Could you check a few things on this model? Use its own coordinates, in mm. Face numbers are marked on the shaded views. A direction names the side the tool comes from. Coordinates: 2 decimals unless noted, no trailing zeros. Write each loop counter-clockwise with the first axis right and the second up, starting at its lowest first coordinate (ties: lowest second). Pieces come first, ordered by that corner, then holes. Notation, with made-up numbers: (14, 37) - (19, 37) arc R25 cw to (19, 55) - close; hole circle Ø1 at (20, -34). An arc over 180 degrees is marked (long way). Answer as a JSON object with one key per item and string values. Group by question number.
1) Please list where these lines run through material, in increasing order: line 1 along Y through (x, z) = (2.5, 0.25); line 2 along X through (y, z) = (-1.9, -0.3); line 3 along X through (y, z) = (2.1, -1.4).
2) On a 3-axis mill with a long thin cutter (end or side, diameter ignored), from which of +Z, -Z, +X, -X, +Y, -Y can I reach the whole of each face in a straight line? I mean the marked faces 1 and 2. Say none if no direction works.
3) If we section it at A-A (x = 3.5): Write out the boundary of the cut face in (y, z).
4) Will these pins go through, and if not, where does the flat tip stop? pin 1 Ø1 at (x, z) = (3.5, -2) entering from +Y; pin 2 Ø3 at (x, z) = (3.5, 1.5) entering from -Y; pin 3 Ø3 at (x, z) = (3.5, 1) entering from +Y; pin 4 Ø1 at (x, y) = (3, 0) entering from -Z.
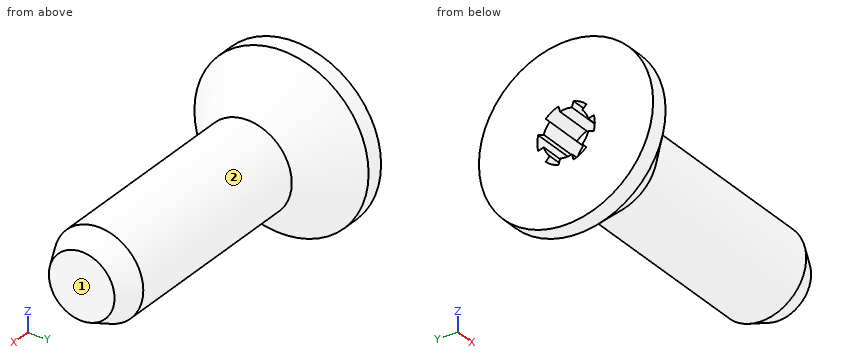
Autodesk Inventor part; units mm, degrees
ref_plane "Work Plane1" through (66.6877, 0, 0) normal (0, 0, -1) x (1, 0, 0)
ref_plane "YZ Plane" through (0, 0, 0) normal (1, 0, 0) x (0, 1, 0)
ref_plane "XZ Plane" through (0, 0, 0) normal (0, 1, 0) x (-1, 0, 0)
sketch "Szkic1" plane through (0, 0, 0) normal (0, 0, 1) x (1, 0, 0)
  line L0 (9.525, 0) -> (9.525, 1.4224)
  line L1 (9.525, 1.4224) -> (2.1082, 1.4224)
  line L2 (0, 2.7686) -> (0, 0.9144)
  line L3 (0, 0.9144) -> (1.397, 0.9144)
  line L4 (1.397, 0.9144) -> (1.9249, 0)
  line L5 (1.9249, 0) -> (9.525, 0)
  line L6 (0, 2.7686) -> (0.5596, 2.7686)
  line L7 (0.5596, 2.7686) -> (2.1082, 1.4224)
  line L8 (-1.905, 0) -> (11.43, 0)
  line L9 (0, -0.5537) -> (0, 3.3223)
  dimension "d0" = 9.525
  dimension "d1" = 1.397
  dimension "d2" = 2.8448
  dimension "d3" = 2.1082
  dimension "d4" = 41
  dimension "d5" = 1.8288
  dimension "d6" = 60
  dimension "d7" = 5.5372
revolve "Bryła" add sketch "Szkic1" angle 360 about axis through (1.9249, 0, 0) along (1, 0, 0) contours L5 L4 L3 L2 L6 L7 L1 L0
sketch "Szkic2" plane through (0, 0, 0) normal (-1, 0, 0) x (0, 0, 1)
  circle A0 centre (0, 0) radius 2.7686
  circle A1 centre (0, 0) radius 0.9144
  line L0 (0.7066, 0.1893) -> (0.8832, 0.2367)
  line L1 (0.7066, -0.1893) -> (0.8832, -0.2367)
  arc A2 (0.7066, -0.1893) -> (0.7066, 0.1893) centre (0, 0) ccw
  arc A3 (0.8832, -0.2367) -> (0.8832, 0.2367) centre (0, 0) ccw
  line L2 (0, -3.876) -> (0, 3.876)
  line L3 (-3.876, 0) -> (3.876, 0)
  line L4 (0.7066, 0.1893) -> (0, 0) construction
  line L5 (0, 0) -> (0.7066, -0.1893) construction
  line L6 (0.1893, 0.7066) -> (0.2367, 0.8832)
  line L7 (0.5173, 0.5173) -> (0.6466, 0.6466)
  arc A4 (0.5173, 0.5173) -> (0.1893, 0.7066) centre (0, 0) ccw
  arc A5 (0.6466, 0.6466) -> (0.2367, 0.8832) centre (0, 0) ccw
  line L8 (-0.5173, 0.5173) -> (-0.6466, 0.6466)
  line L9 (-0.1893, 0.7066) -> (-0.2367, 0.8832)
  arc A6 (-0.1893, 0.7066) -> (-0.5173, 0.5173) centre (0, 0) ccw
  arc A7 (-0.2367, 0.8832) -> (-0.6466, 0.6466) centre (0, 0) ccw
  line L10 (-0.7066, -0.1893) -> (-0.8832, -0.2367)
  line L11 (-0.7066, 0.1893) -> (-0.8832, 0.2367)
  arc A8 (-0.7066, 0.1893) -> (-0.7066, -0.1893) centre (0, 0) ccw
  arc A9 (-0.8832, 0.2367) -> (-0.8832, -0.2367) centre (0, 0) ccw
  line L12 (-0.1893, -0.7066) -> (-0.2367, -0.8832)
  line L13 (-0.5173, -0.5173) -> (-0.6466, -0.6466)
  arc A10 (-0.5173, -0.5173) -> (-0.1893, -0.7066) centre (0, 0) ccw
  arc A11 (-0.6466, -0.6466) -> (-0.2367, -0.8832) centre (0, 0) ccw
  line L14 (0.5173, -0.5173) -> (0.6466, -0.6466)
  line L15 (0.1893, -0.7066) -> (0.2367, -0.8832)
  arc A12 (0.1893, -0.7066) -> (0.5173, -0.5173) centre (0, 0) ccw
  arc A13 (0.2367, -0.8832) -> (0.6466, -0.6466) centre (0, 0) ccw
  dimension "d8" = 1.463
  dimension "d9" = 1.8288
  dimension "d10" = 15
  dimension "d11" = 15
  dimension "d22" = 360
extrude "Szczelina" add sketch "Szkic2" against normal up to next contours L3 A2 L0 A1 | A1 L1 A2 L3 | L3 A8 L10 A1 | A1 L11 A8 L3 | A1 L7 A4 L6 | L9 A6 L8 A1 | A1 L13 A10 L12 | L15 A12 L14 A1
thread "Gwint"
chamfer "Faza1" distance 0.3785 distance2 0.7569 1 edges at (9.525, -1.4224, 0) measured on face at (9.525, -0.1427, 0.3949)
ref_plane "Work Plane1" through (66.6877, 0, 0) normal (0, 0, -1) x (1, 0, 0)
equation "\"d0\" = NLG"
equation "\"d1\" = INTI"
equation "\"d2\" = GD"
equation "\"d3\" = KOH"
equation "\"d4\" = 0.5 * SEWI"
equation "\"d5\" = SW"
equation "\"d7\" = KOD"
equation "\"d8\" = 0.8 * SW"
equation "\"d9\" = SW"
equation "\"d15\" = GEL"
equation "\"d17\" = -0.5 * SPD + 0.5 * GD"
equation "\"d18\" = GUL"
equation "\"NLG\" = 9.525"
equation "\"SW\" = 1.8288"
equation "\"INTI\" = 1.397"
equation "\"GEL\" = 5.8293"
equation "\"KOH\" = 2.1082"
equation "\"KOD\" = 5.5372"
equation "\"GUL\" = 0.75692"
equation "\"SPD\" = 2.08788"
equation "\"GD\" = NND"
equation "\"SEWI\" = 82deg"
equation "\"TOA\" = 30deg"
equation "\"GD1\" = SPD"
equation "\"EPV\" = 3.74448"
equation "\"THREADDIA\" = 2.8448"
equation "\"BDM\" = NND"
equation "\"NND\" = 2.8448"
equation "\"GAL\" = 1.5875"
equation "\"E0\" = 1.155 * SW"
properties part number "ANSI B18.3 - 4-40 UNC x 0,375" material "Stal, miękka"
Here are the results:
{
 "1": {"line 1": "y = -1.4 to 1.4", "line 2": "x = 0 to 1.53", "line 3": "x = 0 to 0.84"},
 "2": {"face 1": "+Z, -Z, +X, +Y, -Y", "face 2": "+X"},
 "3": {"outline": "circle Ø2.84 at (0, 0)"},
 "4": {"pin 1": "passes through", "pin 2": "stops at y = -1.42", "pin 3": "stops at y = 1.42", "pin 4": "stops at z = -1.42"}
}
